Input: part model. Units: mm. Frame: model coordinates. A direction names the side the tool comes from. Give positions to 0.01 mm unless a question says otherwise; leave off trailing zeros. Loops run counter-clockwise (first coordinate to the right, second up) from the corner with the lowest first, then second, coordinate; pieces in that order, holes last. Notation, with made-up numbers: (-25, -15.75) -> (-16, -15.75) arc R34 cw to (-16, 18.25) -> close; hole circle Ø4 at (0, -3.5). An arc over 180 degrees is marked (long way). Use CSV: the item, a comma, the result in double quotes.
```python
from build123d import *

# Parameters (mm, degrees)
F1_DEPTH = 11.3
F2_R     = 3
F3_R     = 2.25
F4_DEPTH = 2.5
F6_DEPTH = 25


# Not quite as in the source:
# - a feature names something its author has since deleted; it is built from what else it names


with BuildPart() as f1:
    # F0 (on Top) → F1 (new body)
    with BuildSketch(Plane.XY):
        Polygon((0, 22.1), (0, 0), (19, 0), (19, -5.2), (21, -5.2), (22, 0), (22, 8.1), (26.6, 8.1), (26.6, 22.1), (22, 22.1), (21, 27.3), (19, 27.3), (19, 22.1), (10, 22.1), (10, 28.1), (6, 28.1), (6, 22.1), align=None)
    extrude(amount=F1_DEPTH)

    # F2
    f2_edges = [f1.edges().sort_by_distance(p)[0] for p in [
        (24.3, 8.1, 0),
        (24.3, 8.1, 11.3),
        (24.3, 22.1, 11.3),
        (24.3, 22.1, 0),
    ]]
    fillet(f2_edges, radius=F2_R)

    # F3 (on face) → F4 (join)
    with BuildSketch(Plane.YZ.offset(26.6)):
        with Locations((16.1, 5.65)):
            Circle(F3_R)
    extrude(amount=F4_DEPTH)

    # F5 (on face) → F6 (cut)
    with BuildSketch(Plane(origin=(19, 0, 0), x_dir=(0, -1, 0), z_dir=(-1, 0, 0))):
        with BuildLine():
            Line((5.2, 4.55), (5.2, 6.75))
            ThreePointArc((5.2, 6.75), (1.8625525219, 5.65), (5.2, 4.55))
        make_face()
        with BuildLine():
            ThreePointArc((-27.3, 4.55), (-25.2334488328, 3.8929744119), (-23.9625525219, 5.65))
            ThreePointArc((-23.9625525219, 5.65), (-25.2334488328, 7.4070255881), (-27.3, 6.75))
            Line((-27.3, 6.75), (-27.3, 4.55))
        make_face()
    extrude(amount=-F6_DEPTH, mode=Mode.SUBTRACT)


solid = f1.part
```
1) Section query D-D (y = 8.5). Return loops of the section in (x, z).
From the geometry:
outline,"(0, 0) -> (22, 0) -> (22, 1.5) -> (26.6, 1.5) -> (26.6, 9.8) -> (22, 9.8) -> (22, 11.3) -> (0, 11.3) -> close"
2) Mould query, pull axis X, two halves, no side actions, for faces 6 (the cylindrical face through (24.33, 8.96, 10.4)), 7 (the flat face through (0, 11, 6)), 8 (the flat face through (19, 23.6, 5.6)). Classes: pulls with the +X half, pulls with the -X half, needs draft (parallel to the pull), parting line crosses it, or undercut.
From the geometry:
face 6,"needs draft"
face 7,"pulls with the -X half"
face 8,"undercut"
3) Section query C-C (z = 10.25). Return loops of the section in (x, y), then the cut area to 3 significant figures.
From the geometry:
outline,"(0, 0) -> (19, 0) -> (19, -5.2) -> (21, -5.2) -> (22, 0) -> (22, 8.82) -> (26.6, 8.82) -> (26.6, 21.38) -> (22.14, 21.38) -> (21, 27.3) -> (19, 27.3) -> (19, 22.1) -> (10, 22.1) -> (10, 28.1) -> (6, 28.1) -> (6, 22.1) -> (0, 22.1) -> close"
area,"594 mm^2"
4) Section query B-B (x = 20.25). Return loops of the section in (y, z), then the cut area to 3 significant figures.
From the geometry:
outline,"(-5.2, 0) -> (27.3, 0) -> (27.3, 4.55) arc R1.85 cw (long way) to (27.3, 6.75) -> (27.3, 11.3) -> (-5.2, 11.3) -> (-5.2, 6.75) arc R1.85 cw (long way) to (-5.2, 4.55) -> close"
area,"347 mm^2"
5) Section query A-A (y = 16.1). Return loops of the section in (x, z), then the cut area to 3 significant figures.
From the geometry:
outline,"(0, 0) -> (26.6, 0) -> (26.6, 3.4) -> (29.1, 3.4) -> (29.1, 7.9) -> (26.6, 7.9) -> (26.6, 11.3) -> (0, 11.3) -> close"
area,"312 mm^2"
6) Contact query for flat-ended pins moving along their axis: pin 1 (2 mm diameter, centred on y = 12.5, z = 1.5, fed in from -X); pin 2 (3.5 mm diameter, centred on y = 5.5, z = 4.5, fed in from +X); pin 3 (1.5 mm diameter, centred on x = 18, z = 2, fed in from +Y); pin 4 (1.6 mm diameter, centred on x = 19.5, z = 3, fed in from +Y). Output: stop coordinate, or through.
From the geometry:
pin 1,"stops at x = 0"
pin 2,"stops at x = 22"
pin 3,"stops at y = 22.1"
pin 4,"stops at y = 27.3"
7) Ray query, line 1 (X direction, y = 10.5, z = 3.25); line 2 (X direction, y = 4.5, z = 2); line 3 (Y direction, x = 20.8, z = 5.65). Return the intervals inside material, ascending.
From the geometry:
line 1,"x = 0 to 26.6"
line 2,"x = 0 to 22"
line 3,"y = -1.86 to 23.96"
8) Reachability of faces 1 (the cylindrical face through (24.27, 21.24, 0.9)), 2 (the flat face through (24, 8.1, 6)), 3 (the flat face through (24, 22.1, 6)), 4 (the flat face through (3, 22.1, 6)), 5 (the cylindrical face through (27.833, 18.246, 6.326)) from +Z, -Z, +X, -X, +Y, -Y: full face, straight path, thin tool, end or side. Return the list, or none.
From the geometry:
face 1,"-Z, +X, +Y"
face 2,"+Z, -Z, +X, -Y"
face 3,"+Z, -Z, +X, +Y"
face 4,"+Z, -Z, -X, +Y"
face 5,"+X"
